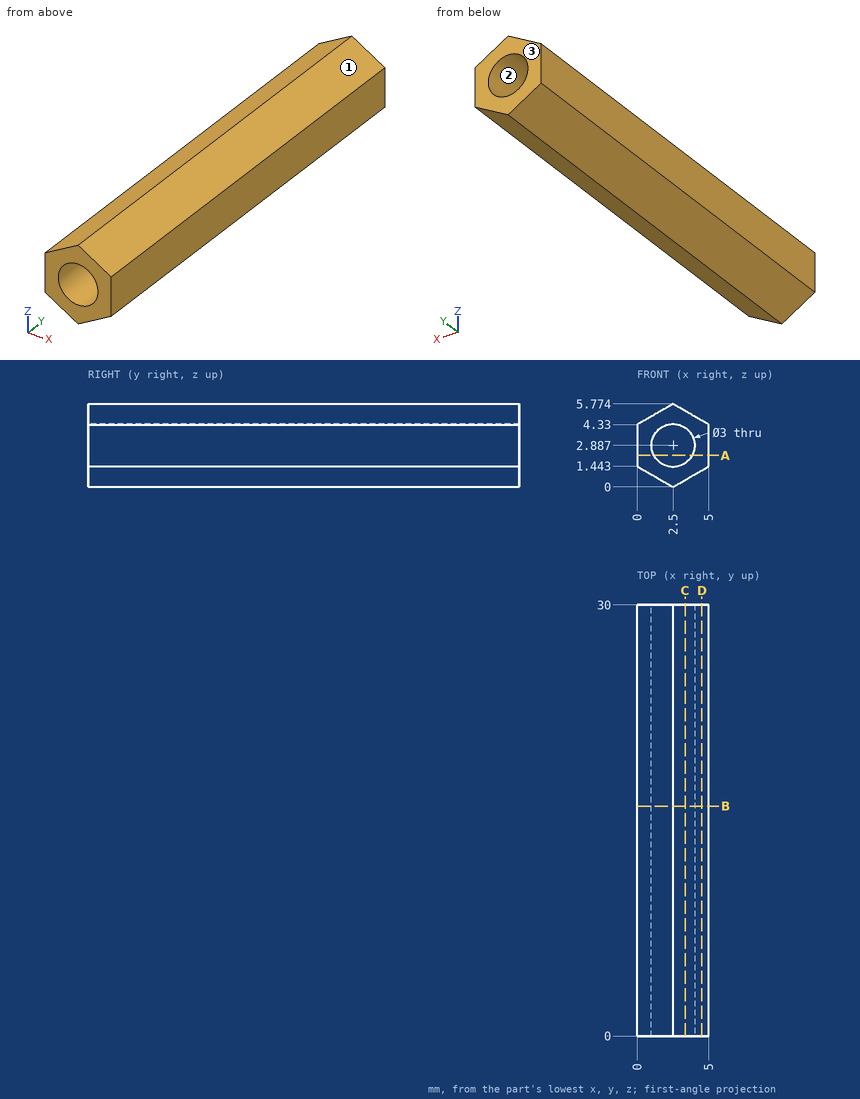
Design review of the part shown in the three views and the two pictorial views. Dimensions are in mm from the part's minimum x, y and z. Give positions to 0.01 mm unless a question says otherwise; leave off trailing zeros. Write each loop counter-clockwise with the first axis right and the second up, starting at its lowest first coordinate (ties: lowest second). Pieces come first, ordered by that corner, then holes.
Item 1: Wall thickness on probe 1 along X at (y, z) = (21.25, 2.95); probe 2 along X at (y, z) = (2.25, 2.2) (1 decimal); probe 3 along Z at (x, y) = (3.4, 18.5) (1 decimal): over which ranges is each line inside the solid? List them lowest first.
Item 2: Take a section at A-A (z = 2.2). Give the boundary of the cut face in (x, y).
Item 3: Take a section at B-B (y = 16). Give the boundary of the cut face in (x, z), and give its area (3 significant figures).
Item 4: Take a section at C-C (x = 3.35). Give the boundary of the cut face in (y, z).
Item 5: Insertion check: P1, Ø2, axis at y = 13.5, z = 4.5, coming from the -X side. The pin has a flat end and moves straight along its axis. Give the tip position at first contact, or say it passes through.
Item 6: The part is to be moulded in two halves that separate along X. For the marked faces 1, 2 and 3, say which applies: +X half, -X half, draft (parallel to the pull), parting line (faces both ways), or undercut.
Item 7: Take a section at D-D (x = 4.5). Give the boundary of the cut face in (y, z) (1 decimal).
Established:
1. probe 1: x = 0 to 1, 4 to 5
1. probe 2: x = 0 to 1.2, 3.8 to 5
1. probe 3: z = 0.5 to 1.7, 4.1 to 5.3
2. outline: (0, 0) - (1.17, 0) - (1.17, 30) - (0, 30) - close; (3.83, 0) - (5, 0) - (5, 30) - (3.83, 30) - close
3. outline: (0, 1.44) - (2.5, 0) - (5, 1.44) - (5, 4.33) - (2.5, 5.77) - (0, 4.33) - close; hole circle Ø3 at (2.5, 2.89)
3. area: 14.6 mm2
4. outline: (0, 0.49) - (30, 0.49) - (30, 1.65) - (0, 1.65) - close; (0, 4.12) - (30, 4.12) - (30, 5.28) - (0, 5.28) - close
5. P1: stops at x = 0
6. face 1: +X half
6. face 2: undercut
6. face 3: draft
7. outline: (0, 1.2) - (30, 1.2) - (30, 4.6) - (0, 4.6) - close
